Geometry check sheet. Reference: the model listing, model coordinates, mm. A direction names the side the tool comes from. Round coordinates to 2 decimals unless told otherwise and drop trailing zeros. Order: outer loops, then holes, each group sorted by start corner. A loop starts at its lowest first (then second) coordinate and runs counter-clockwise, first axis right, second up.
(1) Sectioned sample at D-D (z = 7.75). Record the boundary of the cut face in (x, y), plus the area to 3 significant figures.
(2) Sectioned sample at B-B (x = 13). Record the boundary of the cut face in (y, z), plus the area to 3 significant figures.
(3) Sectioned sample at C-C (y = -9.75). Record the boundary of the cut face in (x, z), plus the area to 3 significant figures.
(4) Sectioned sample at A-A (y = -11.75). Record the boundary of the cut face in (x, z).
(5) Go/stop test with flat-tipped pins: pin 1 (5 mm diameter, centred on x = 2.5, y = -12, fed in from -Z); pin 2 (2 mm diameter, centred on x = 4.5, z = 19, fed in from -Y). Record where each tip stops, or that it passes through.
(6) Material ranges on line 1 along X through (y, z) = (-13, 8.5); line 2 along Y through (x, z) = (19.5, 15); line 3 along Y through (x, z) = (22.5, 11.5), recorded low to high.
(7) Set-up check for faces 5 (the face through (19, -10.1, 13)), 6 (the face through (0, -5, 13)), 7 (the face through (7.7, -9.5, 26.5)): record each of +Z, -Z, +X, -X, +Y, -Y from which the full face is reachable in a straight line by a thin tool's end or side.
(8) Release check for a two-part mould opening along Y. For faces 1 (the face through (23, -15.3, 13)), 2 (the face through (19, -8.9, 13)), 3 (the face through (4, -8.9, 13)), 4 (the face through (0.8, -13, 13)) record: +Y half, -Y half, draft (parallel to the pull), parting line (faces both ways), or undercut.
from build123d import *

# Parameters (mm, degrees)
EXTRUDE_1_DEPTH = 26.5
SKETCH_2_W      = 2
SKETCH_2_H      = 26.5
EXTRUDE_2_DEPTH = 5.2


with BuildPart() as part:
    # 草图1 → 凸台-拉伸1 (new body)
    with BuildSketch(Plane.XY):
        Polygon((-1.2, 1.2), (24.2, 1.2), (24.2, -10.1), (15.7, -10.1), (15.7, -15.3), (7.3, -15.3), (7.3, -10.1), (-1.2, -10.1), align=None)
        Polygon((0, 0), (23, 0), (23, -8.9), (14.5, -8.9), (14.5, -14.1), (8.5, -14.1), (8.5, -8.9), (0, -8.9), align=None, mode=Mode.SUBTRACT)
    extrude(amount=EXTRUDE_1_DEPTH)

    # 草图2 → 凸台-拉伸2 (add)
    with BuildSketch(Plane.XZ.offset(10.1)):
        with Locations((-0.2, 13.25)):
            Rectangle(SKETCH_2_W, SKETCH_2_H)
        with Locations((23.2, 13.25)):
            Rectangle(SKETCH_2_W, SKETCH_2_H)
    extrude(amount=EXTRUDE_2_DEPTH)


solid = part.part
Answer below:
1. outline: (-1.2, -15.3) - (0.8, -15.3) - (0.8, -10.1) - (7.3, -10.1) - (7.3, -15.3) - (15.7, -15.3) - (15.7, -10.1) - (22.2, -10.1) - (22.2, -15.3) - (24.2, -15.3) - (24.2, 1.2) - (-1.2, 1.2) - close; hole (0, -8.9) - (8.5, -8.9) - (8.5, -14.1) - (14.5, -14.1) - (14.5, -8.9) - (23, -8.9) - (23, 0) - (0, 0) - close
1. area: 116 mm2
2. outline: (-15.3, 0) - (-14.1, 0) - (-14.1, 26.5) - (-15.3, 26.5) - close; (0, 0) - (1.2, 0) - (1.2, 26.5) - (0, 26.5) - close
2. area: 63.6 mm2
3. outline: (-1.2, 0) - (8.5, 0) - (8.5, 26.5) - (-1.2, 26.5) - close; (14.5, 0) - (24.2, 0) - (24.2, 26.5) - (14.5, 26.5) - close
3. area: 514 mm2
4. outline: (-1.2, 0) - (0.8, 0) - (0.8, 26.5) - (-1.2, 26.5) - close; (7.3, 0) - (8.5, 0) - (8.5, 26.5) - (7.3, 26.5) - close; (14.5, 0) - (15.7, 0) - (15.7, 26.5) - (14.5, 26.5) - close; (22.2, 0) - (24.2, 0) - (24.2, 26.5) - (22.2, 26.5) - close
5. pin 1: stops at z = 0
5. pin 2: stops at y = -10.1
6. line 1: x = -1.2 to 0.8, 7.3 to 8.5, 14.5 to 15.7, 22.2 to 24.2
6. line 2: y = -10.1 to -8.9, 0 to 1.2
6. line 3: y = -15.3 to -8.9, 0 to 1.2
7. face 5: +Z, -Z, -Y
7. face 6: +Z, -Z
7. face 7: +Z, +X, -X, +Y, -Y
8. face 1: -Y half
8. face 2: undercut
8. face 3: undercut
8. face 4: draft
